from build123d import *

# Parameters (mm, degrees)
SKETCH1_W                  = 61.658
SKETCH1_H                  = 76.028
BOSS_EXTRUDE1_DEPTH        = 15.8
SKETCH3_W                  = 58.158
SKETCH3_H                  = 70.528
CUT_EXTRUDE2_DEPTH         = 14.8
FILLET1_R                  = 7
FILLET2_R                  = 7
FILLET3_R                  = 7
SKETCH4_W                  = 1.75
SKETCH4_H                  = 16.5
CUT_EXTRUDE3_SWITCH_DEPTH  = 12
SKETCH5_W                  = 1.75
SKETCH5_H                  = 9
CUT_EXTRUDE4_USB_DEPTH     = 12
SKETCH6_R                  = 8.5
CUT_EXTRUDE4_SONIC_DEPTH   = 2.75
SKETCH7_W                  = 37.258
SKETCH7_H                  = 35.8
CUT_EXTRUDE5_LCDMAIN_DEPTH = 1
SKETCH8_W                  = 37.258
SKETCH8_H                  = 6.8
CUT_EXTRUDE6_LCDNOTI_DEPTH = 1
FILLET4_R                  = 5
FILLET5_R                  = 2
FILLET6_R                  = 3.4


with BuildPart() as part:
    # Sketch1 → Boss-Extrude1 (new body)
    with BuildSketch(Plane.XY):
        with Locations((30.829, 38.014)):
            Rectangle(SKETCH1_W, SKETCH1_H)
    extrude(amount=BOSS_EXTRUDE1_DEPTH)

    # Sketch3 → Cut-Extrude2 (cut)
    with BuildSketch(Plane.XY.offset(15.8)):
        with Locations((30.829, 38.014)):
            Rectangle(SKETCH3_W, SKETCH3_H)
    extrude(amount=-CUT_EXTRUDE2_DEPTH, mode=Mode.SUBTRACT)

    # Fillet1
    fillet1_edges = [part.edges().sort_by_distance(p)[0] for p in [
        (61.658, 76.028, 7.9),
    ]]
    fillet(fillet1_edges, radius=FILLET1_R)

    # Fillet2
    fillet2_edges = [part.edges().sort_by_distance(p)[0] for p in [
        (1.75, 73.278, 8.4),
        (61.658, 0, 7.9),
        (0, 0, 7.9),
    ]]
    fillet(fillet2_edges, radius=FILLET2_R)

    # Fillet3
    fillet3_edges = [part.edges().sort_by_distance(p)[0] for p in [
        (1.75, 2.75, 8.4),
        (59.908, 73.278, 8.4),
        (59.908, 2.75, 8.4),
        (0, 76.028, 7.9),
    ]]
    fillet(fillet3_edges, radius=FILLET3_R)

    # Sketch4 → Cut-Extrude3_switch (cut)
    with BuildSketch(Plane.XY.offset(15.8)):
        with Locations((0.875, 50.194669907)):
            Rectangle(SKETCH4_W, SKETCH4_H)
    extrude(amount=-CUT_EXTRUDE3_SWITCH_DEPTH, mode=Mode.SUBTRACT)

    # Sketch5 → Cut-Extrude4_usb (cut)
    with BuildSketch(Plane.XY.offset(15.8)):
        with Locations((0.875, 27.643981113)):
            Rectangle(SKETCH5_W, SKETCH5_H)
    extrude(amount=-CUT_EXTRUDE4_USB_DEPTH, mode=Mode.SUBTRACT)

    # Sketch6 → Cut-Extrude4_sonic (cut)
    with BuildSketch(Plane(origin=(0, 76.028, 0), x_dir=(1, 0, 0), z_dir=(0, 1, 0))):
        with Locations((29.25, -15.8)):
            Circle(SKETCH6_R)
    extrude(amount=-CUT_EXTRUDE4_SONIC_DEPTH, mode=Mode.SUBTRACT)

    # Sketch7 → Cut-Extrude5_LcdMain (cut)
    with BuildSketch(Plane(origin=(0, 0, 0), x_dir=(-1, 0, 0), z_dir=(0, 0, -1))):
        with Locations((-30.829, 45.928)):
            Rectangle(SKETCH7_W, SKETCH7_H)
    extrude(amount=-CUT_EXTRUDE5_LCDMAIN_DEPTH, mode=Mode.SUBTRACT)

    # Sketch8 → Cut-Extrude6_LcdNoti (cut)
    with BuildSketch(Plane(origin=(0, 0, 0), x_dir=(-1, 0, 0), z_dir=(0, 0, -1))):
        with Locations((-30.829, 15.6)):
            Rectangle(SKETCH8_W, SKETCH8_H)
    extrude(amount=-CUT_EXTRUDE6_LCDNOTI_DEPTH, mode=Mode.SUBTRACT)

    # Fillet4
    fillet4_edges = [part.edges().sort_by_distance(p)[0] for p in [
        (49.458, 63.828, 0.5),
        (12.2, 63.828, 0.5),
    ]]
    fillet(fillet4_edges, radius=FILLET4_R)

    # Fillet5
    fillet5_edges = [part.edges().sort_by_distance(p)[0] for p in [
        (49.458, 28.028, 0.5),
        (12.2, 28.028, 0.5),
    ]]
    fillet(fillet5_edges, radius=FILLET5_R)

    # Fillet6
    fillet6_edges = [part.edges().sort_by_distance(p)[0] for p in [
        (12.2, 12.2, 0.5),
        (12.2, 19, 0.5),
        (49.458, 19, 0.5),
        (49.458, 12.2, 0.5),
    ]]
    fillet(fillet6_edges, radius=FILLET6_R - 0.0001)  # a hair under: the kernel refuses the full size


solid = part.part
Build history of the part. All positions in model axes, mm. A direction names the side the tool comes from. Coordinates: 2 decimals unless noted, no trailing zeros. Order: outer loops, then holes, each group sorted by start corner. A loop starts at its lowest first (then second) coordinate and runs counter-clockwise, first axis right, second up. Notation, with made-up numbers: (-7.75, 37) -> (23.25, 37) arc R17 ccw to (23.25, 54) -> close; hole circle Ø5 at (68, 10.5). An arc over 180 degrees is marked (long way). One line per item, written item: value.
(1) Slice it at D-D, the plane z = 11. List the corners of the cut face in (x, y), plus the area to 3 significant figures.
Checked values:
outline: (0, 7) arc R7 ccw to (7, 0) -> (54.66, 0) arc R7 ccw to (61.66, 7) -> (61.66, 69.03) arc R7 ccw to (54.66, 76.03) -> (36.26, 76.03) -> (36.26, 73.28) -> (52.91, 73.28) arc R7 cw to (59.91, 66.28) -> (59.91, 9.75) arc R7 cw to (52.91, 2.75) -> (8.75, 2.75) arc R7 cw to (1.75, 9.75) -> (1.75, 23.14) -> (0, 23.14) -> close; (0, 32.14) -> (1.75, 32.14) -> (1.75, 41.94) -> (0, 41.94) -> close; (0, 58.44) -> (1.75, 58.44) -> (1.75, 66.28) arc R7 cw to (8.75, 73.28) -> (22.24, 73.28) -> (22.24, 76.03) -> (7, 76.03) arc R7 ccw to (0, 69.03) -> close
area: 503 mm2
(2) Slice it at A-A, the plane x = 29.25. List the corners of the cut face in (y, z).
Checked values:
outline: (0, 0) -> (12.2, 0) -> (12.2, 1) -> (2.75, 1) -> (2.75, 15.8) -> (0, 15.8) -> close; (19, 0) -> (28.03, 0) -> (28.03, 1) -> (19, 1) -> close; (63.83, 0) -> (76.03, 0) -> (76.03, 7.3) -> (73.28, 7.3) -> (73.28, 1) -> (63.83, 1) -> close
(3) Tool access for faces 5 (the cylindrical face through (48.032, 62.324, 0.507)), 6 (the flat face through (1, 28, 3.8)), 7 (the cylindrical face through (2.105, 74.032, 8.011)), 8 (the flat face through (6, 73, 15.8)), 9 (the cylindrical face through (57.803, 71.282, 8.296)): list every direction of +Z, -Z, +X, -X, +Y, -Y with a clear straight run to the whole face (end or side of a thin tool).
Checked values:
face 5: +Z, -Z
face 6: +Z, -X
face 7: +Z, -Z, -X, +Y
face 8: +Z, +X, -X, +Y, -Y
face 9: +Z
(4) Slice it at C-C, the plane y = 34. List the corners of the cut face in (x, z).
Checked values:
outline: (0, 0) -> (12.2, 0) -> (12.2, 1) -> (1.75, 1) -> (1.75, 15.8) -> (0, 15.8) -> close; (49.46, 0) -> (61.66, 0) -> (61.66, 15.8) -> (59.91, 15.8) -> (59.91, 1) -> (49.46, 1) -> close
(5) Mould opens along Y. For faces 1 (the cylindrical face through (59.662, 2.105, 8.011)), 2 (the cylindrical face through (12.8, 28.6, 0.5)), 3 (the flat face through (30, 22, 0)), 4 (the flat face through (30, 76.028, 6)) say: pulls with the +Y half, pulls with the -Y half, needs draft (parallel to the pull), parting line crosses it, or undercut.
Checked values:
face 1: pulls with the -Y half
face 2: undercut
face 3: needs draft
face 4: pulls with the +Y half
(6) Probe line 1 (Y direction, x = 37, z = 1.25); line 2 (X direction, y = 59, z = 6); line 3 (X direction, y = 50.5, z = 14.5). List the from-to ranges inside material, lowest first. Write a range as [from, to].
Checked values:
line 1: [0, 2.75], [73.28, 76.03]
line 2: [0, 1.75], [59.91, 61.66]
line 3: [59.91, 61.66]
(7) Slice it at B-B, the plane z = 4.75. List the corners of the cut face in (x, y).
Checked values:
outline: (0, 7) arc R7 ccw to (7, 0) -> (54.66, 0) arc R7 ccw to (61.66, 7) -> (61.66, 69.03) arc R7 ccw to (54.66, 76.03) -> (7, 76.03) arc R7 ccw to (0, 69.03) -> (0, 58.44) -> (1.75, 58.44) -> (1.75, 66.28) arc R7 cw to (8.75, 73.28) -> (52.91, 73.28) arc R7 cw to (59.91, 66.28) -> (59.91, 9.75) arc R7 cw to (52.91, 2.75) -> (8.75, 2.75) arc R7 cw to (1.75, 9.75) -> (1.75, 23.14) -> (0, 23.14) -> close; (0, 32.14) -> (1.75, 32.14) -> (1.75, 41.94) -> (0, 41.94) -> close
(8) Drop flat-ended pins along their axis: pin 1 Ø0.5 at (x, z) = (1, 10.5) entering from -Y; pin 2 Ø1.9 at (x, y) = (0.5, 47) entering from +Z; pin 3 Ø5 at (x, y) = (15, 42) entering from -Z; pin 4 Ø0.9 at (x, z) = (0.5, 10) entering from +Y. Give the stop position or say it passes through.
Checked values:
pin 1: y = 3.01
pin 2: z = 3.8
pin 3: through
pin 4: y = 72.55
